Answer from the drawing. Dimensions are ordinates in mm from the lowest x, y and z of the part. A direction names the side the tool comes from. Give positions to 0.01 mm unless a question says otherwise; leave off trailing zeros. Order: outer loops, then holes, each group sorted by start corner. A loop starts at its lowest first (then second) coordinate and runs counter-clockwise, first axis right, second up.
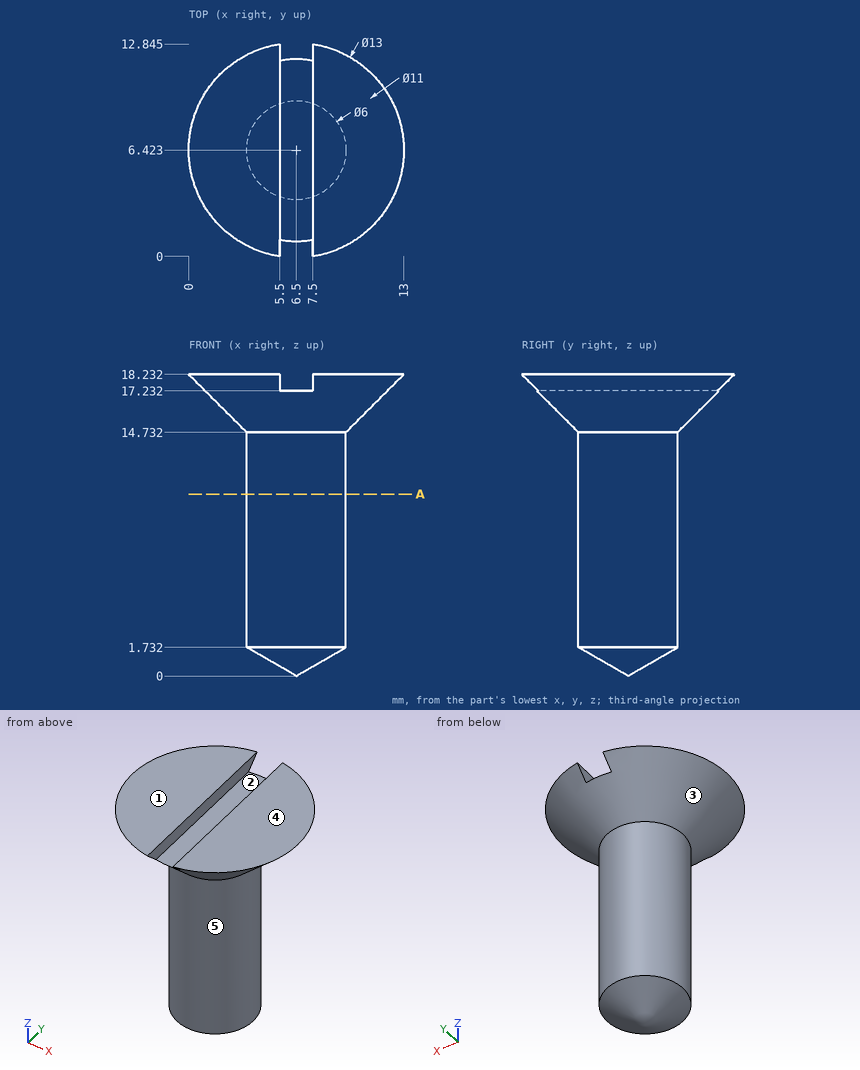
1. Given P1, Ø1, axis at y = 11.5, z = 15.5, coming from the -X side; P2, Ø3, axis at y = 6, z = 9, coming from the +X side; P3, Ø0.8, axis at y = 7, z = 18, coming from the -X side (1 decimal); P4, Ø1.5, axis at y = 6, z = 16, coming from the -X side, each flat-ended and moving along its own axis, determine where each tip first touches the part or whether it passes through.
Findings below:
P1: passes through
P2: stops at x = 9.5
P3: stops at x = 0
P4: stops at x = 1.5
2. Straight lines are drawn through the part: probe 1 along X at (y, z) = (6.5, 14.25); probe 2 along Y at (x, z) = (9.5, 15.25) (1 decimal); probe 3 along Z at (x, y) = (12, 8) (1 decimal). For each, find the intervals that lie inside material, in ascending order.
Findings below:
probe 1: x = 3.5 to 9.5
probe 2: y = 4.6 to 8.3
probe 3: z = 17.5 to 18.2
3. Which of the six approach directions +Z, -Z, +X, -X, +Y, -Y give full straight-line access (tool end or side, diameter ignored) to the marked faces 4 and 5?
Findings below:
face 4: +Z, +X, -X, +Y, -Y
face 5: -Z
4. The mould has two halves that part along X. Classify the marked faces 1, 2 and 3: pulls with the +X half, pulls with the -X half, needs draft (parallel to the pull), parting line crosses it, or undercut.
Findings below:
face 1: needs draft
face 2: undercut
face 3: parting line crosses it
5. The part is cut by section A-A (z = 11). Write down the section's boundary in (x, y).
Findings below:
outline: circle Ø6 at (6.5, 6.42)
